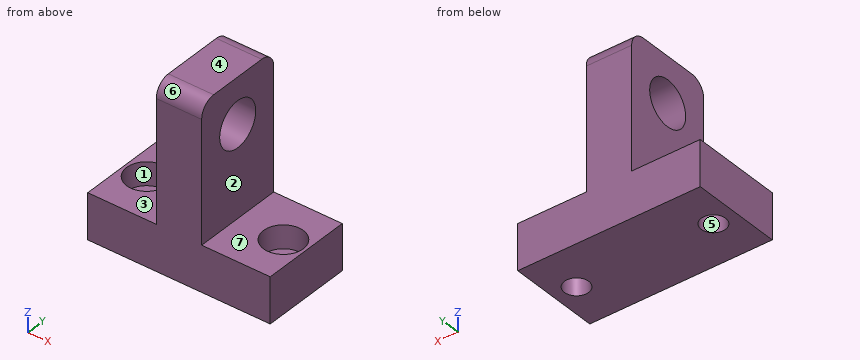
```python
from build123d import *

# Parameters (mm, degrees)
SKETCH1_W                = 38.1
SKETCH1_H                = 19.05
SKETCH1_R                = 2.53365
BOSS_EXTRUDE1_DEPTH      = 9.525
SKETCH2_R                = 4.16052
CUT_EXTRUDE1_DEPTH       = 4.826
BOSS_EXTRUDE2_DEPTH      = 4.7371
BOSS_EXTRUDE2_DEPTH_BACK = 4.7371
SKETCH3_W                = 28.575
SKETCH3_H                = 19.05
SKETCH3_R                = 4.7625
FILLET1_R                = 3.175


with BuildPart() as part:
    # Sketch1 → Boss-Extrude1 (new body)
    with BuildSketch(Plane.XY):
        Rectangle(SKETCH1_W, SKETCH1_H)
        with Locations(Location((-14.2875, 0, 0), (0, 0, 180))):
            Circle(SKETCH1_R, mode=Mode.SUBTRACT)
        with Locations(Location((14.2875, 0, 0), (0, 0, 180))):
            Circle(SKETCH1_R, mode=Mode.SUBTRACT)
    extrude(amount=BOSS_EXTRUDE1_DEPTH)

    # Sketch2 → Cut-Extrude1 (cut)
    with BuildSketch(Plane.XY.offset(9.525)):
        with Locations((-14.2875, 0)):
            Circle(SKETCH2_R)
        with Locations((14.2875, 0)):
            Circle(SKETCH2_R)
    extrude(amount=-CUT_EXTRUDE1_DEPTH, mode=Mode.SUBTRACT)

    # Sketch3 → Boss-Extrude2 (add, two sides: drawn at the far end of the back side and taken through both)
    with BuildSketch(Plane(origin=(0, 0, 0), x_dir=(0, 0, -1), z_dir=(1, 0, 0)).offset(-BOSS_EXTRUDE2_DEPTH_BACK)):
        with Locations((-23.8125, 0)):
            Rectangle(SKETCH3_W, SKETCH3_H)
        with Locations(Location((-28.575, 0, 0), (0, 0, 180))):
            Circle(SKETCH3_R, mode=Mode.SUBTRACT)
    extrude(amount=BOSS_EXTRUDE2_DEPTH + BOSS_EXTRUDE2_DEPTH_BACK)

    # Fillet1
    fillet1_edges = [part.edges().sort_by_distance(p)[0] for p in [
        (0, -9.525, 38.1),
        (0, 9.525, 38.1),
    ]]
    fillet(fillet1_edges, radius=FILLET1_R)


solid = part.part
```
For this review, take the finished solid that the model builds, in its own axes (mm). Face numbers are marked on the shaded views. A direction names the side the tool comes from. Give positions to 0.01 mm unless a question says otherwise; leave off trailing zeros. Write each loop counter-clockwise with the first axis right and the second up, starting at its lowest first coordinate (ties: lowest second). Pieces come first, ordered by that corner, then holes. Notation, with made-up numbers: M -21,36.25 L 2,36.25 A15 cw 2,63.25 Z; hole C 73,37.25 d8. An arc over 180 degrees is marked long. Answer as a JSON object with one key per item and string values. Group by question number.
Item 1: Consider section A-A on y = 0. Count the separate pieces of the cut face and the enclosed holes in it, plus the area to 3 significant figures.
Item 2: Draft analysis for pull direction Y (two halves, no side actions). For the marked faces 5, 6 and 7, state which applies: +Y half, -Y half, draft (parallel to the pull), parting line (faces both ways), or undercut.
Item 3: Consider section C-C on x = 15. Write out the cut boundary in (y, z) (3 decimals).
Item 4: Tool access review of the marked faces 1, 2, 3 and 4: name each direction out of +Z, -Z, +X, -X, +Y, -Y from which nothing blocks a thin tool from reaching the whole face with its end or side.
Item 5: For probe 1 along Y at (x, z) = (-14, 5.5) (3 decimals); probe 2 along X at (y, z) = (2.5, 9); probe 3 along Z at (x, y) = (-14.5, 5.5) (3 decimals), list the stretches that pass through material, from the lowest coordinate up. Write a range as [from, to].
Item 6: Consider section D-D on y = -5.75. Write out the cut boundary in (x, z) (3 decimals), plus the area to 3 significant figures.
Item 7: For pin 1 Ø9.5 at (y, z) = (-1.5, 20) entering from -X; pin 2 Ø8 at (y, z) = (-1.5, 24.5) entering from +X; pin 3 Ø4 at (x, y) = (-15.5, -0.5) entering from +Z, all flat-tipped, find the tip position at first contact; note any pin that passes through.
Check result:
{
 "1": {"separate pieces": "4", "enclosed holes": "0", "area": "415 mm^2"},
 "2": {"face 5": "undercut", "face 6": "-Y half", "face 7": "draft"},
 "3": {"outline": "M -9.525,0 L -2.431,0 L -2.431,4.699 L -4.099,4.699 L -4.099,9.525 L -9.525,9.525 Z; M 2.431,0 L 9.525,0 L 9.525,9.525 L 4.099,9.525 L 4.099,4.699 L 2.431,4.699 Z"},
 "4": {"face 1": "+Z", "face 2": "+Z, +X, +Y, -Y", "face 3": "+Z, -X, +Y, -Y", "face 4": "+Z, +X, -X, +Y, -Y"},
 "5": {"probe 1": "y = [-9.525, -4.151], [4.151, 9.525]", "probe 2": "x = [-19.05, -17.61], [-10.96, 10.96], [17.61, 19.05]", "probe 3": "z = [0, 9.525]"},
 "6": {"outline": "M -19.05,0 L 19.05,0 L 19.05,9.525 L 4.737,9.525 L 4.737,38.1 L -4.737,38.1 L -4.737,9.525 L -19.05,9.525 Z", "area": "634 mm^2"},
 "7": {"pin 1": "stops at x = -4.74", "pin 2": "stops at x = 4.74", "pin 3": "stops at z = 4.7"}
}
